Read the model definition and answer for the solid it produces. Units are mm, in the model's axes. A direction names the side the tool comes from. Give positions to 0.01 mm unless a question says otherwise; leave off trailing zeros. Loops run counter-clockwise (first coordinate to the right, second up) from the corner with the lowest first, then second, coordinate; pieces in that order, holes last. Notation, with made-up numbers: (11.25, 57) - (27.25, 57) arc R25 cw to (27.25, 82) - close; hole circle Ø9 at (54, 26). An arc over 180 degrees is marked (long way). Write item = value, one per line.
```python
from build123d import *

# Parameters (mm, degrees)
F0_R     = 22.110067
F1_DEPTH = 7.62
F2_DEPTH = 25.4
F4_DEPTH = 3.302


with BuildPart() as f1:
    # F0 (on Top) → F1 (new body)
    with BuildSketch(Plane.XY):
        with BuildLine():
            ThreePointArc((18.473424, 5.673436), (28.299088, 17.017198), (31.836316, 31.601869))
            ThreePointArc((31.836316, 31.601869), (-14.584671, 59.900956), (-18.473424, 5.673436))
            ThreePointArc((-18.473424, 5.673436), (0, -0.234447), (18.473424, 5.673436))
        make_face()
        with Locations((0, 31.601869)):
            Circle(F0_R, mode=Mode.SUBTRACT)
        with BuildLine():
            ThreePointArc((18.473424, 5.673436), (0, -0.234447), (-18.473424, 5.673436))
            Line((-18.473424, 5.673436), (-18.473424, -35.552085))
            Line((-18.473424, -35.552085), (0, -35.552085))
            Line((0, -35.552085), (18.473424, -35.552085))
            Line((18.473424, -35.552085), (18.473424, 5.673436))
        make_face()
    extrude(amount=-F1_DEPTH)

    # F0 (on Top) → F2 (join)
    with BuildSketch(Plane.XY):
        with BuildLine():
            ThreePointArc((18.473424, 5.673436), (28.299088, 17.017198), (31.836316, 31.601869))
            ThreePointArc((31.836316, 31.601869), (-14.584671, 59.900956), (-18.473424, 5.673436))
            ThreePointArc((-18.473424, 5.673436), (0, -0.234447), (18.473424, 5.673436))
        make_face()
        with Locations((0, 31.601869)):
            Circle(F0_R, mode=Mode.SUBTRACT)
    extrude(amount=F2_DEPTH)

    # F3 (on Right) → F4 (join, symmetric)
    with BuildSketch(Plane.YZ):
        Polygon((0, 24.508493), (-28.300449, 0), (3.349552, 0), (3.349552, 24.508493), align=None)
    extrude(amount=F4_DEPTH, both=True)


solid = f1.part
```
1) A cutting plane is placed at D-D on x = -16. Determine the outline of the cut face in (y, z), then the cut area to 3 significant figures.
Output:
outline = (-35.55, -7.62) - (16.34, -7.62) - (16.34, 25.4) - (4.08, 25.4) - (4.08, 0) - (-35.55, 0) - close; (46.86, -7.62) - (59.13, -7.62) - (59.13, 25.4) - (46.86, 25.4) - close
area = 1,110 mm²
2) A cutting plane is placed at A-A on x = 15. Determine the outline of the cut face in (y, z).
Output:
outline = (-35.55, -7.62) - (15.36, -7.62) - (15.36, 25.4) - (3.52, 25.4) - (3.52, 0) - (-35.55, 0) - close; (47.85, -7.62) - (59.68, -7.62) - (59.68, 25.4) - (47.85, 25.4) - close
3) The mould has two halves that part along Y. Classify faces 4 (the face through (-4.793, 10.018, 8.659)), 5 (the face through (0, -35.552, -4)), 6 (the face through (18.473, -15, -4)): pulls with the +Y half, pulls with the -Y half, needs draft (parallel to the pull), parting line crosses it, or undercut.
Output:
face_4 = undercut
face_5 = pulls with the -Y half
face_6 = needs draft
4) A tool of negligible diameter and unlimited length cuts with its end or side. For faces 1 (the face through (-18.473, -15, -4)), 2 (the face through (4, -15, 0)), 3 (the face through (-3.302, -8, 7)), from which of +Z, -Z, +X, -X, +Y, -Y can it reach the whole face along a straight path? Write none if from no direction.
Output:
face_1 = +Z, -Z, -X, -Y
face_2 = +Z, -Y
face_3 = +Z, -X, -Y
5) Find the intervals of material crossed by probe 1 along X at (y, z) = (-21, 1); probe 2 along Z at (x, y) = (4.5, -20.5); probe 3 along Y at (x, z) = (0, 5), in increasing order.
Output:
probe_1 = -3.3 to 3.3
probe_2 = -7.62 to 0
probe_3 = -22.53 to 9.49, 53.71 to 63.44
6) A cutting plane is placed at B-B on y = 50. Determine the outline of the cut face in (x, z).
Output:
outline = (-25.98, -7.62) - (-12.26, -7.62) - (-12.26, 25.4) - (-25.98, 25.4) - close; (12.26, -7.62) - (25.98, -7.62) - (25.98, 25.4) - (12.26, 25.4) - close
7) A cutting plane is placed at C-C on z = 15. Determine the outline of the cut face in (x, y), then the cut area to 3 significant figures.
Output:
outline = (-18.47, 5.67) arc R31.84 ccw to (-3.3, -0.06) - (-3.3, -10.98) - (3.3, -10.98) - (3.3, -0.06) arc R31.84 ccw to (18.47, 5.67) arc R31.84 ccw to (31.84, 31.6) arc R31.84 ccw (long way) to start; hole circle Ø44.22 at (0, 31.6)
area = 1,720 mm²
8) Each of these flat-tipped pins is pushed along its axis until it touches: P1, Ø6, axis at y = -13.5, z = -4.5, coming from the +X side; P2, Ø12, axis at y = -12, z = 17.5, coming from the -X side; P3, Ø4, axis at x = -17.5, z = 4.5, coming from the -Y side. Where does it stop, or does it pass through?
Output:
P1 = 18.47
P2 = -3.3
P3 = 3.79
